Here's the drawing with two shaded views (mm, measured from the low corner). I have some questions. Round coordinates to 2 decimals unless told otherwise and drop trailing zeros. Loops run counter-clockwise (first coordinate to the right, second up) from the corner with the lowest first, then second, coordinate; pieces in that order, holes last. Notation, with made-up numbers: M -36,57.5 L 7,57.5 A18 ccw 7,85.5 Z; hole C 73.5,64.5 d1. An arc over 180 degrees is marked long. Answer as CSV lines item,"result".
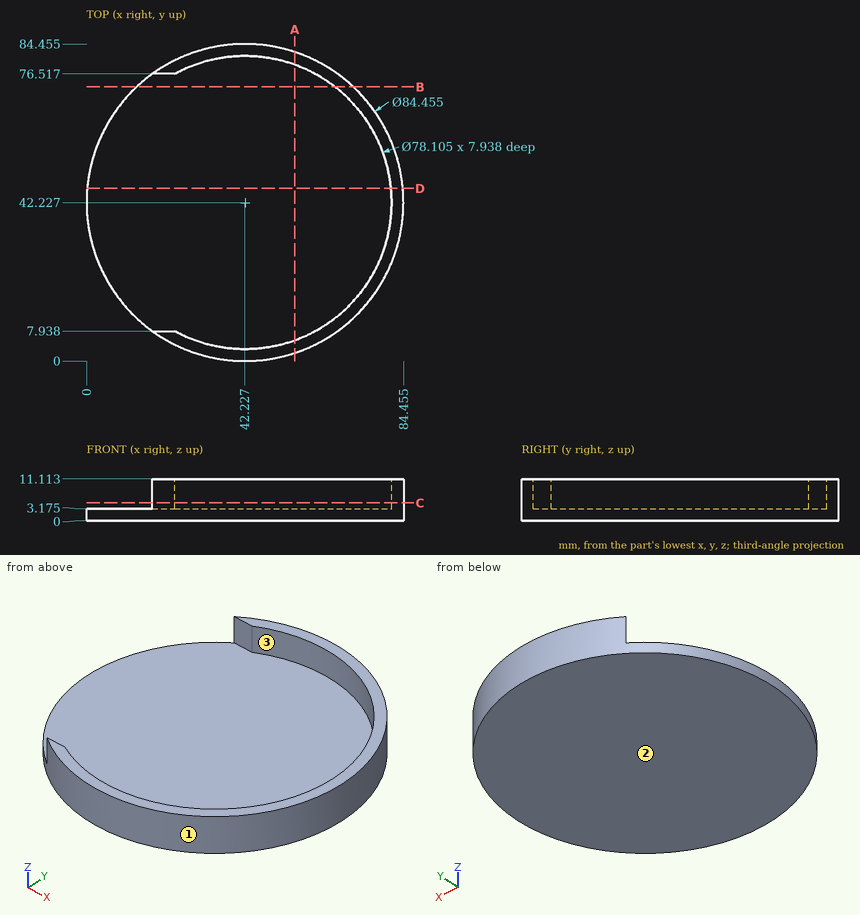
1. I want a section at C-C, the plane z = 4.75. Please give me the cut outline in (x, y) (1 decimal).
Evaluation:
outline,"M 17.6,7.9 A42.2 ccw long 17.6,76.5 L 23.5,76.5 A39.1 cw long 23.5,7.9 Z"
2. I want a section at A-A, the plane x = 55.5. Please give me the cut outline in (y, z) (1 decimal), and give its area (3 significant figures).
Evaluation:
outline,"M 2.1,0 L 82.3,0 L 82.3,11.1 L 79,11.1 L 79,3.2 L 5.5,3.2 L 5.5,11.1 L 2.1,11.1 Z"
area,"308 mm²"
3. We'd pull the mould along X, two halves only. Please class the marked faces 1, 2 and 3: pulls with the +X half, pulls with the -X half, needs draft (parallel to the pull), parting line crosses it, or undercut.
Evaluation:
face 1,"parting line crosses it"
face 2,"needs draft"
face 3,"undercut"
4. For P1, Ø6, axis at x = 20, z = 2.5, coming from the -Y side; P2, Ø4, axis at y = 67, z = 4.5, coming from the +X side; P3, Ø8, axis at x = 40, y = 46.5, coming from the +Z side (1 decimal), each with a flat end and sliding along its axis, tell me the tip position at first contact or that it passes through.
Evaluation:
P1,"stops at y = 4.63"
P2,"stops at x = 77.79"
P3,"stops at z = 3.2"
5. If I drill on line 1 (Z direction, x = 32, y = 45) (1 decimal); line 2 (Y direction, x = 69, z = 5) (1 decimal); line 3 (Y direction, x = 26.5, z = 6.75) (1 decimal), over which ranges is the centre line in solid material (lowest first)? Write a range as [from, to].
Evaluation:
line 1,"z = [0, 3.2]"
line 2,"y = [9.6, 13.8], [70.7, 74.9]"
line 3,"y = [3, 6.5], [78, 81.4]"
6. I want a section at B-B, the plane y = 73. Please give me the cut outline in (x, z) (1 decimal), and give its area (3 significant figures).
Evaluation:
outline,"M 13.3,0 L 71.1,0 L 71.1,11.1 L 66.3,11.1 L 66.3,3.2 L 13.3,3.2 Z"
area,"222 mm²"
7. I want a section at D-D, the plane y = 46. Please give me the cut outline in (x, z) (1 decimal).
Evaluation:
outline,"M 0.2,0 L 84.3,0 L 84.3,11.1 L 81.1,11.1 L 81.1,3.2 L 0.2,3.2 Z"
